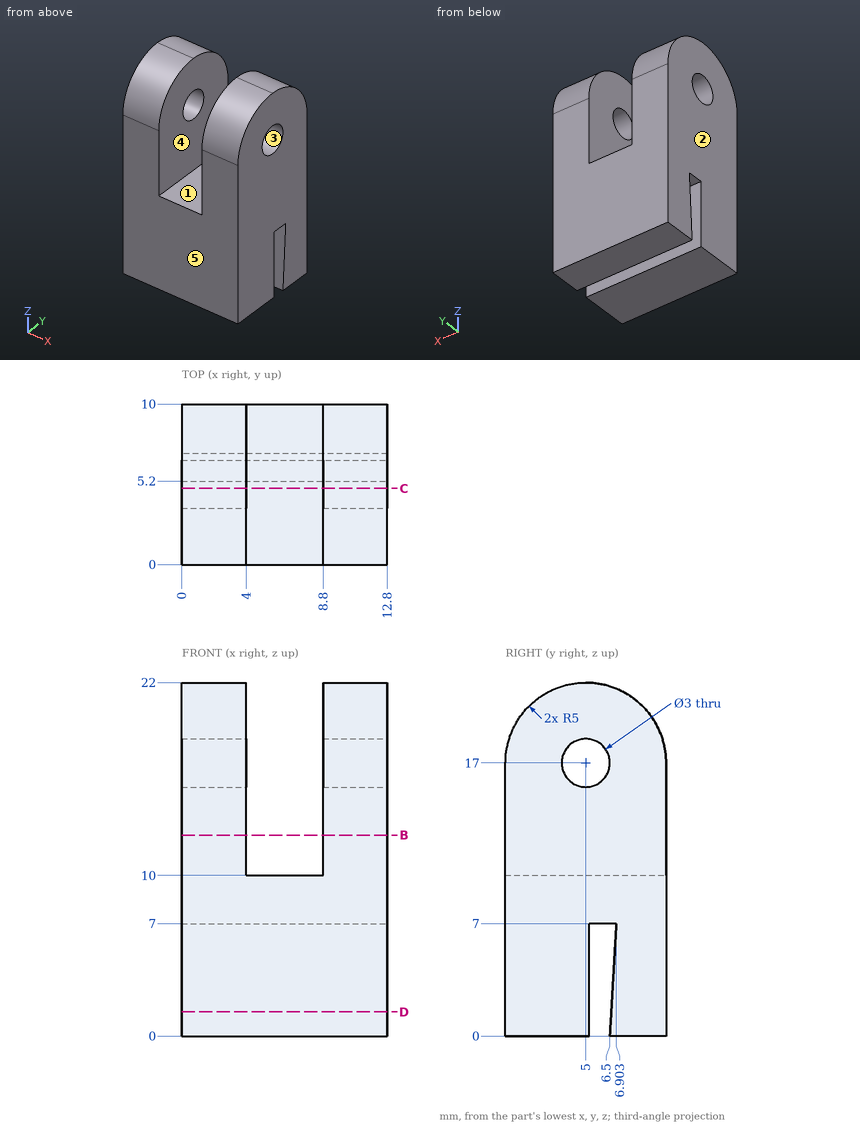
Design review of the part shown in the three views and the two pictorial views. Dimensions are in mm from the part's minimum x, y and z. A direction names the side the tool comes from. Give positions to 0.01 mm unless a question says otherwise; leave off trailing zeros. Order: outer loops, then holes, each group sorted by start corner. A loop starts at its lowest first (then second) coordinate and runs counter-clockwise, first axis right, second up. Notation, with made-up numbers: M 29,-23.75 L 83,-23.75 A35 cw 83,11.25 Z; hole C -27.75,86 d8. An arc over 180 degrees is marked long. Answer in a Markdown table with one row per item. Add a question column.
(1) For the marked faces 4 and 5, list the 3-axis set-ups (+Z, -Z, +X, -X, +Y, -Y) from which the entire face can be reached by the end or side of a thin tool; tool diameter is ignored.
(2) Consider section D-D on z = 1.5. State the section outline as (x, y) points.
(3) Wall thickness on probe 1 along X at (y, z) = (8.25, 18.5); probe 2 along Y at (x, z) = (2.4, 17); probe 3 along Z at (x, y) = (4.75, 2.5): over which ranges is each line inside the solid? List them lowest first. Write a range as [from, to].
(4) Consider section B-B on z = 12.5. State the section outline as (x, y) points.
(5) Mouldability with a two-part tool opening along X and no side actions: class the marked faces 1, 2 and 3 as +X half, -X half, draft (parallel to the pull), parting line (faces both ways), or undercut.
(6) Consider section C-C on y = 4.75. State the section outline as (x, z) points, and give its area (3 significant figures).
Evaluation:
| question | item | result |
|---|---|---|
| 1 | face 4 | +Z, +Y, -Y |
| 1 | face 5 | +Z, -Z, +X, -X, -Y |
| 2 | outline | M 0,0 L 12.8,0 L 12.8,5.2 L 0,5.2 Z; M 0,6.59 L 12.8,6.59 L 12.8,10 L 0,10 Z |
| 3 | probe 1 | x = [0, 4], [8.8, 12.8] |
| 3 | probe 2 | y = [0, 3.5], [6.5, 10] |
| 3 | probe 3 | z = [0, 10] |
| 4 | outline | M 0,0 L 4,0 L 4,10 L 0,10 Z; M 8.8,0 L 12.8,0 L 12.8,10 L 8.8,10 Z |
| 5 | face 1 | undercut |
| 5 | face 2 | -X half |
| 5 | face 3 | draft |
| 6 | outline | M 0,0 L 12.8,0 L 12.8,15.52 L 8.8,15.52 L 8.8,10 L 4,10 L 4,15.52 L 0,15.52 Z; M 0,18.48 L 4,18.48 L 4,21.99 L 0,21.99 Z; M 8.8,18.48 L 12.8,18.48 L 12.8,21.99 L 8.8,21.99 Z |
| 6 | area | 200 mm^2 |
